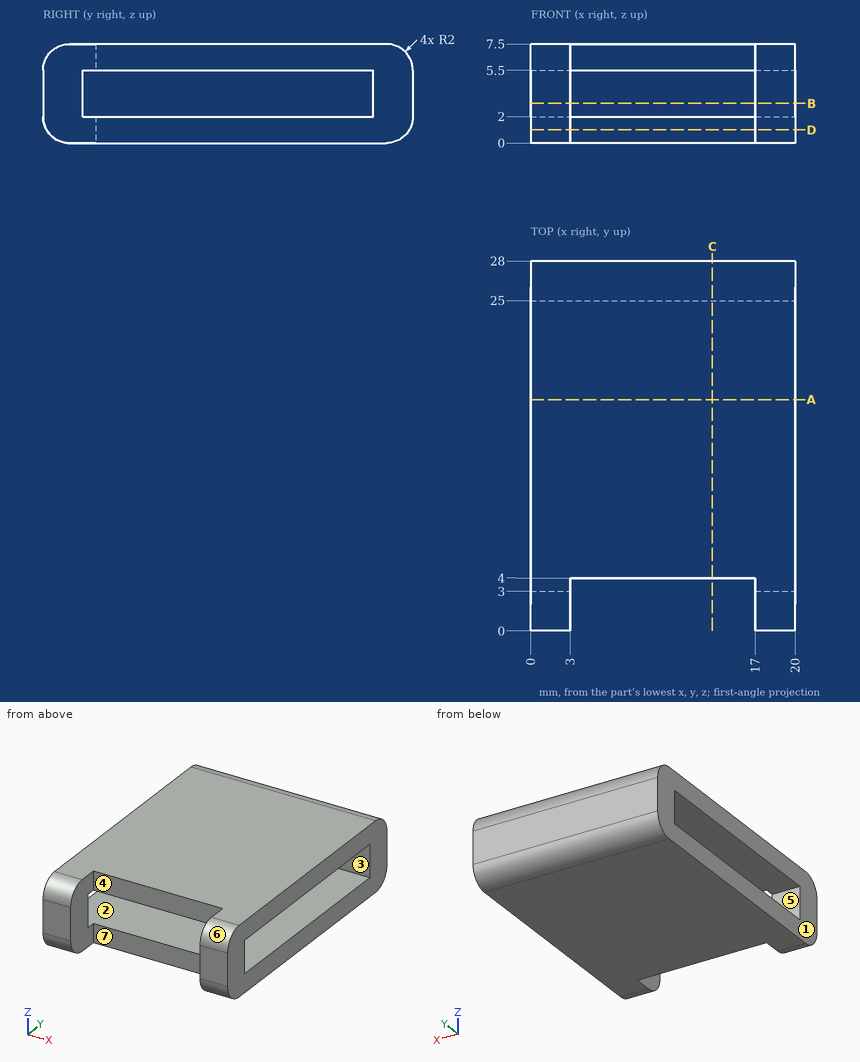
Check sheet for the drawn part. Datum: minimum x, y, z corner. Units: mm. A direction names the side the tool comes from. Coordinates: 2 decimals unless noted, no trailing zeros. Write each loop counter-clockwise with the first axis right and the second up, starting at its lowest first coordinate (ties: lowest second). Pieces come first, ordered by that corner, then holes. Notation, with made-up numbers: (77, 0) - (105, 0) arc R16 ccw to (105, 13) - close; hole circle Ø6 at (5, 21.5). An arc over 180 degrees is marked (long way). Answer as a JSON object with one key per item and string values.
(1) Thickness scan on line 1 along Y through (x, z) = (17.75, 4.75); line 2 along Z through (x, y) = (18.75, 11.5); line 3 along X through (y, z) = (3.25, 6). Record the ranges inside material, lowest first.
Report:
{"line 1": "0 to 3, 25 to 28", "line 2": "0 to 2, 5.5 to 7.5", "line 3": "0 to 3, 17 to 20"}
(2) Cross-section at B-B on z = 3. Record the cut outline in (x, y), plus the area to 3 significant figures.
Report:
{"outline": "(0, 0) - (3, 0) - (3, 3) - (0, 3) - close; (0, 25) - (20, 25) - (20, 28) - (0, 28) - close; (17, 0) - (20, 0) - (20, 3) - (17, 3) - close", "area": "78.0 mm^2"}
(3) Mould release check, pull along Y, two halves, no side actions. Record for the marked faces 1, 2, 3 and 4: pulls with the +Y half, pulls with the -Y half, needs draft (parallel to the pull), parting line crosses it, or undercut.
Report:
{"face 1": "needs draft", "face 2": "undercut", "face 3": "undercut", "face 4": "pulls with the -Y half"}
(4) Cross-section at C-C on x = 13.75. Record the cut outline in (y, z).
Report:
{"outline": "(4, 0) - (26, 0) arc R2 ccw to (28, 2) - (28, 5.5) arc R2 ccw to (26, 7.5) - (4, 7.5) - (4, 5.5) - (25, 5.5) - (25, 2) - (4, 2) - close"}
(5) Cross-section at A-A on y = 17.5. Record the cut outline in (x, z).
Report:
{"outline": "(0, 0) - (20, 0) - (20, 2) - (0, 2) - close; (0, 5.5) - (20, 5.5) - (20, 7.5) - (0, 7.5) - close"}
(6) Gauge pin test, flat ends, axial feed: pin 1 Ø1 at (x, z) = (5.5, 3) entering from -Y; pin 2 Ø1 at (x, z) = (7.5, 1) entering from -Y. Record the tip position at first contact, or that the pin passes through.
Report:
{"pin 1": "y = 25", "pin 2": "y = 4"}
(7) Cross-section at D-D on z = 1. Record the cut outline in (x, y), plus the area to 3 significant figures.
Report:
{"outline": "(0, 0.27) - (3, 0.27) - (3, 4) - (17, 4) - (17, 0.27) - (20, 0.27) - (20, 27.73) - (0, 27.73) - close", "area": "497 mm^2"}
(8) Tool access check on the marked faces 5, 6 and 7. Record the directions out of +Z, -Z, +X, -X, +Y, -Y that give a thin tool (end or side, any length) a straight path to the whole face; none if there is none.
Report:
{"face 5": "+X, -X", "face 6": "+Z, +X, -X, -Y", "face 7": "+Z, -Z, -Y"}
